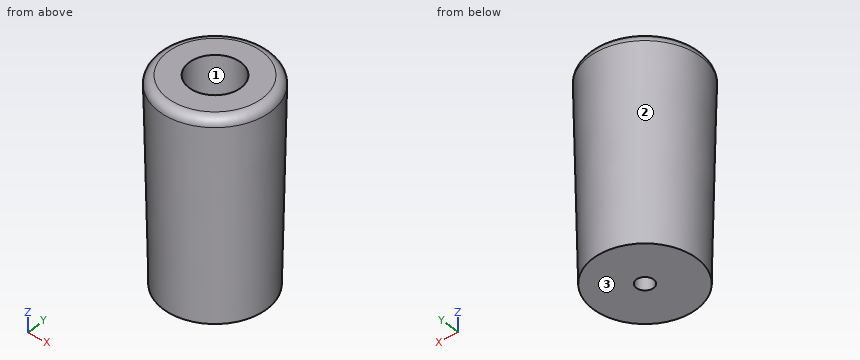
from build123d import *

# Parameters (mm, degrees)
F2_R     = 0.5
F3_R     = 1.5
F4_DEPTH = 10
F5_R     = 0.5
F6_DEPTH = 2


with BuildPart() as f1:
    # F0 (on Front) → F1 (revolve)
    with BuildSketch(Plane.XZ):
        Polygon((0, 6.186947), (0, -5.563053), (3, -5.563053), (3.25, 6.186947), align=None)
    revolve(axis=Axis((0, 0, 0.311947), (0, 0, 1)))

    # F2
    f2_edges = [f1.edges().sort_by_distance(p)[0] for p in [
        (-3.25, 0, 6.186947),
    ]]
    fillet(f2_edges, radius=F2_R)

    # F3 (on face) → F4 (cut)
    with BuildSketch(Plane.XY.offset(6.186947)):
        Circle(F3_R)
    extrude(amount=-F4_DEPTH, mode=Mode.SUBTRACT)

    # F5 (on face) → F6 (cut)
    with BuildSketch(Plane(origin=(0, 0, -5.563053), x_dir=(1, 0, 0), z_dir=(0, 0, -1))):
        Circle(F5_R)
    extrude(amount=-F6_DEPTH, mode=Mode.SUBTRACT)


solid = f1.part
Verification items for the finished model (mm, model axes). Face numbers are marked on the shaded views. Coordinates: 2 decimals unless noted, no trailing zeros. Order: outer loops, then holes, each group sorted by start corner. A loop starts at its lowest first (then second) coordinate and runs counter-clockwise, first axis right, second up. Notation, with made-up numbers: (51.25, 19.5) -> (88.25, 19.5) arc R9 cw to (88.25, 25.5) -> close; hole circle Ø1 at (54, 88.5). An arc over 180 degrees is marked (long way). Put each result on its own line as item: value. Start each with the question number.
1. Cross-section at A-A, the plane y = 0. Record the boundary of the cut face in (x, z), then the cut area to 3 significant figures.
2. Go/stop test with flat-tipped pins: pin 1 Ø2.5 at (x, y) = (-0.5, 0.5) entering from +Z; pin 2 Ø2.5 at (x, y) = (0, 0) entering from +Z; pin 3 Ø3 at (y, z) = (0, 2.5) entering from -X; pin 4 Ø3 at (x, z) = (1, -1.5) entering from +Y. Record where each tip stops, or that it passes through.
3. Cross-section at D-D, the plane z = -1.5. Record the boundary of the cut face in (x, y), then the cut area to 3 significant figures.
4. Material ranges on L1, parallel to Y at x = 0, z = -1.25; L2, parallel to Y at x = 0.5, z = -0.75; L3, parallel to Z at x = 0.5, y = 2.75, recorded low to high. Write a range as [from, to].
5. Cross-section at C-C, the plane z = -4. Record the boundary of the cut face in (x, y).
6. Mould release check, pull along X, two halves, no side actions. Record for the marked faces 1, 2 and 3: released by +X, released by -X, zero draft, split by the parting line, or undercut.
Computed:
1. outline: (-3.24, 5.68) -> (-3, -5.56) -> (-0.5, -5.56) -> (-0.5, -3.81) -> (-1.5, -3.81) -> (-1.5, 6.19) -> (-2.74, 6.19) arc R0.5 ccw to start; (0.5, -5.56) -> (3, -5.56) -> (3.24, 5.68) arc R0.5 ccw to (2.74, 6.19) -> (1.5, 6.19) -> (1.5, -3.81) -> (0.5, -3.81) -> close
1. area: 41.6 mm2
2. pin 1: z = 6.19
2. pin 2: z = -3.81
2. pin 3: x = -3.2
2. pin 4: y = 3.11
3. outline: circle Ø6.17 at (0, 0); hole circle Ø3 at (0, 0)
3. area: 22.9 mm2
4. L1: [-3.09, -1.5], [1.5, 3.09]
4. L2: [-3.06, -1.41], [1.41, 3.06]
4. L3: [-5.56, 6.18]
5. outline: circle Ø6.07 at (0, 0); hole circle Ø1 at (0, 0)
6. face 1: undercut
6. face 2: split by the parting line
6. face 3: zero draft
